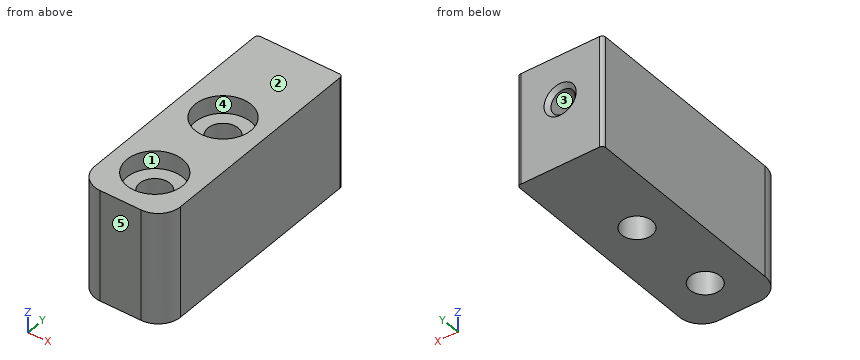
from build123d import *

# Parameters (mm, degrees)
SKETCH1_W                                      = 15.875
SKETCH1_H                                      = 33.3502
BOSS_EXTRUDE1_DEPTH                            = 6.096
CBORE_FOR_8_SOCKET_HEAD_CAP_SCREW1_D           = 4.3053
CBORE_FOR_8_SOCKET_HEAD_CAP_SCREW1_CBORE_D     = 7.9375
CBORE_FOR_8_SOCKET_HEAD_CAP_SCREW1_CBORE_DEPTH = 2.54
F_8_32_TAPPED_HOLE1_D                          = 3.4544
F_8_32_TAPPED_HOLE1_DEPTH                      = 15.24
F_8_32_TAPPED_HOLE1_CSINK_D                    = 4.572
F_8_32_TAPPED_HOLE1_CSINK_ANGLE                = 90
F_8_32_TAPPED_HOLE1_TIP                        = 1.037806461
FILLET1_R                                      = 3.175
FILLET2_R                                      = 0.508


with BuildPart() as part:
    # Sketch1 → Boss-Extrude1 (new, symmetric)
    with BuildSketch(Plane(origin=(0, 0, 0), x_dir=(0, 0, -1), z_dir=(1, 0, 0))):
        with Locations((-7.9375, -16.6751)):
            Rectangle(SKETCH1_W, SKETCH1_H)
    extrude(amount=BOSS_EXTRUDE1_DEPTH, both=True)

    # CBORE for #8 Socket Head Cap Screw1 (through all)
    with Locations(Plane.XY.offset(15.875)):
        with Locations((0, -14.3002), (0, -27.0002)):
            CounterBoreHole(CBORE_FOR_8_SOCKET_HEAD_CAP_SCREW1_D / 2, CBORE_FOR_8_SOCKET_HEAD_CAP_SCREW1_CBORE_D / 2, CBORE_FOR_8_SOCKET_HEAD_CAP_SCREW1_CBORE_DEPTH)

    # #8-32 Tapped Hole1
    with Locations(Plane(origin=(0, 0, 0), x_dir=(-1, 0, 0), z_dir=(0, 1, 0))):
        with Locations((0, 9.525)):
            CounterSinkHole(F_8_32_TAPPED_HOLE1_D / 2, F_8_32_TAPPED_HOLE1_CSINK_D / 2, depth=F_8_32_TAPPED_HOLE1_DEPTH, counter_sink_angle=F_8_32_TAPPED_HOLE1_CSINK_ANGLE)
            with Locations((0, 0, -(F_8_32_TAPPED_HOLE1_DEPTH + F_8_32_TAPPED_HOLE1_TIP / 2))):  # 118° drill point
                Cone(0, F_8_32_TAPPED_HOLE1_D / 2, F_8_32_TAPPED_HOLE1_TIP, mode=Mode.SUBTRACT)

    # Fillet1
    fillet1_edges = [part.edges().sort_by_distance(p)[0] for p in [
        (6.096, -33.3502, 7.9375),
        (-6.096, -33.3502, 7.9375),
    ]]
    fillet(fillet1_edges, radius=FILLET1_R)

    # Fillet2
    fillet2_edges = [part.edges().sort_by_distance(p)[0] for p in [
        (-6.096, 0, 7.9375),
        (6.096, 0, 7.9375),
    ]]
    fillet(fillet2_edges, radius=FILLET2_R)


solid = part.part
Work out the finished part from the listing and answer in its coordinate system (mm). Face numbers are marked on the shaded views. A direction names the side the tool comes from. Round coordinates to 2 decimals unless told otherwise and drop trailing zeros. Write each loop counter-clockwise with the first axis right and the second up, starting at its lowest first coordinate (ties: lowest second). Pieces come first, ordered by that corner, then holes. Notation, with made-up numbers: M -39,-26.5 L -15,-26.5 A35 cw -15,12.5 Z; hole C 76.25,-38 d3. An arc over 180 degrees is marked long. Use a Markdown table: item, result.
1) The part is cut by section C-C on y = -5.5. Give the vertices of the cut face in (x, z) (3 decimals).
Taken from the geometry:
| item | result |
|---|---|
| outline | M -6.096,0 L 6.096,0 L 6.096,15.875 L -6.096,15.875 Z; hole C 0,9.525 d3.454 |
2) The part is cut by section A-A on x = 0. Give the vertices of the cut face in (y, z) (3 decimals), plus the area to 3 significant figures.
Taken from the geometry:
| item | result |
|---|---|
| outline | M -33.35,0 L -29.153,0 L -29.153,13.335 L -30.969,13.335 L -30.969,15.875 L -33.35,15.875 Z; M -24.848,0 L -16.453,0 L -16.453,13.335 L -18.269,13.335 L -18.269,15.875 L -23.031,15.875 L -23.031,13.335 L -24.848,13.335 Z; M -12.148,0 L 0,0 L 0,7.239 L -0.559,7.798 L -12.148,7.798 Z; M -12.148,11.252 L -0.559,11.252 L 0,11.811 L 0,15.875 L -10.331,15.875 L -10.331,13.335 L -12.148,13.335 Z |
| area | 332 mm2 |
3) Consider line 1 (Y direction, x = 0, z = 7.75); line 2 (Y direction, x = 0, z = 13.9); line 3 (X direction, y = -27.5, z = 12.25). Determine where each line is inside the solid, lowest interval first. Write a range as [from, to].
Taken from the geometry:
| item | result |
|---|---|
| line 1 | y = [-33.35, -29.15], [-24.85, -16.45], [-12.15, -0.51] |
| line 2 | y = [-33.35, -30.97], [-23.03, -18.27], [-10.33, 0] |
| line 3 | x = [-6.1, -2.09], [2.09, 6.1] |
4) The part is cut by section D-D on x = -3.5. Give the vertices of the cut face in (y, z) (3 decimals), plus the area to 3 significant figures.
Taken from the geometry:
| item | result |
|---|---|
| outline | M -33.297,0 L 0,0 L 0,15.875 L -12.429,15.875 L -12.429,13.335 L -16.171,13.335 L -16.171,15.875 L -25.129,15.875 L -25.129,13.335 L -28.871,13.335 L -28.871,15.875 L -33.297,15.875 Z |
| area | 510 mm2 |
5) The part is cut by section B-B on z = 5. Give the vertices of the cut face in (x, y) (3 decimals).
Taken from the geometry:
| item | result |
|---|---|
| outline | M -6.096,-30.175 A3.175 ccw -2.921,-33.35 L 2.921,-33.35 A3.175 ccw 6.096,-30.175 L 6.096,-0.508 A0.508 ccw 5.588,0 L -5.588,0 A0.508 ccw -6.096,-0.508 Z; hole C 0,-27 d4.305; hole C 0,-14.3 d4.305 |
6) Determine the mould class of the marked faces 3, 4 and 5 for opening direction Y: pulls with the +Y half, pulls with the -Y half, needs draft (parallel to the pull), parting line crosses it, or undercut.
Taken from the geometry:
| item | result |
|---|---|
| face 3 | needs draft |
| face 4 | undercut |
| face 5 | pulls with the -Y half |
7) A flat-ended cylindrical pin translates along its axis: pin 1 (2.5 mm diameter, centred on x = -2, y = -15, fed in from +Z) (3 decimals). Find the tip coordinate at first contact, or state that the pin passes through.
Taken from the geometry:
| item | result |
|---|---|
| pin 1 | stops at z = 13.335 |
8) Which of the six approach directions +Z, -Z, +X, -X, +Y, -Y give full straight-line access (tool end or side, diameter ignored) to the marked faces 1 and 2?
Taken from the geometry:
| item | result |
|---|---|
| face 1 | +Z |
| face 2 | +Z, +X, -X, +Y, -Y |
